For this review, take the finished solid that the model builds, in its own axes (mm). Face numbers are marked on the shaded views. A direction names the side the tool comes from. Round coordinates to 2 decimals unless told otherwise and drop trailing zeros. Write each loop counter-clockwise with the first axis right and the second up, starting at its lowest first coordinate (ties: lowest second). Pieces come first, ordered by that corner, then holes. Notation, with made-up numbers: (22.5, 83.5) -> (79.5, 83.5) arc R33 ccw to (79.5, 117.5) -> close; hole circle Ø6 at (73, 33.5). An arc over 180 degrees is marked (long way). Write each question's results on one line, items separated by ' | '. Start each with the question number.
Item 1: To check wall thickness, follow line 1 along Y through (x, z) = (12.5, 3.75); line 2 along Y through (x, z) = (97.5, 6); line 3 along Y through (x, z) = (165, 12.5). State the ranges of each line that lie inside material, in increasing order.
Item 2: Tool access review of the marked faces 5 and 6: name each direction out of +Z, -Z, +X, -X, +Y, -Y from which nothing blocks a thin tool from reaching the whole face with its end or side.
Item 3: Add section C-C (y = 10). State the section outline as (x, z) points, plus the area to 3 significant figures.
Item 4: Add section B-B (x = 111.5). State the section outline as (y, z) points, plus the area to 3 significant figures.
Item 5: Add section A-A (z = 14.5). State the section outline as (x, y) points.
Item 6: The part is to be moulded in two halves that separate along Y. For the marked faces 1, 2, 3 and 4, say which applies: +Y half, -Y half, draft (parallel to the pull), parting line (faces both ways), or undercut.
Item 7: Clearance check with flat-ended pins moving along their axes: pin 1 (2.5 mm diameter, centred on x = 12.5, y = -47.5, fed in from -Z); pin 2 (3 mm diameter, centred on x = 15.5, z = 12, fed in from +Y); pin 3 (7.5 mm diameter, centred on x = 13.5, y = -44.5, fed in from +Z); pin 4 (1 mm diameter, centred on x = 159, z = 2.5, fed in from +Y). State where each tip first meets the part, or that it passes through.
from build123d import *

# Parameters (mm, degrees)
PAD_DEPTH       = 18
FILLET_R        = 5
FILLET001_R     = 5
FILLET002_R     = 1
FILLET003_R     = 1
CHAMFER_SIZE    = 7
CHAMFER001_SIZE = 7
SKETCH001_W     = 15
SKETCH001_H     = 15
POCKET_DEPTH    = 10
SKETCH002_R     = 1
POCKET001_DEPTH = 8
SKETCH003_R     = 1
POCKET002_DEPTH = 8


with BuildPart() as part:
    # Sketch → Pad (new body)
    with BuildSketch(Plane.XY):
        Polygon((206.173076, -21.002959), (196.173076, -21.002959), (188.480768, -50), (0, 0), (7.692308, 28.997041), (-10, 28.997041), (-10, -69.999032), (206.173076, -69.999032), align=None)
    extrude(amount=PAD_DEPTH)

    # Fillet
    fillet_edges = [part.edges().sort_by_distance(p)[0] for p in [
        (7.692308, 28.997041, 9),
    ]]
    fillet(fillet_edges, radius=FILLET_R)

    # Fillet001
    fillet001_edges = [part.edges().sort_by_distance(p)[0] for p in [
        (196.173076, -21.002959, 9),
    ]]
    fillet(fillet001_edges, radius=FILLET001_R)

    # Fillet002
    fillet002_edges = [part.edges().sort_by_distance(p)[0] for p in [
        (206.173076, -21.002959, 9),
    ]]
    fillet(fillet002_edges, radius=FILLET002_R)

    # Fillet003
    fillet003_edges = [part.edges().sort_by_distance(p)[0] for p in [
        (-10, 28.997041, 9),
    ]]
    fillet(fillet003_edges, radius=FILLET003_R)

    # Chamfer
    chamfer_edges = [part.edges().sort_by_distance(p)[0] for p in [
        (0, 0, 9),
    ]]
    chamfer(chamfer_edges, length=CHAMFER_SIZE)

    # Chamfer001
    chamfer001_edges = [part.edges().sort_by_distance(p)[0] for p in [
        (188.480768, -50, 9),
    ]]
    chamfer(chamfer001_edges, length=CHAMFER001_SIZE)

    # Sketch001 → Pocket (cut)
    with BuildSketch(Plane.XY.offset(18)):
        with Locations((12.5, -47.499032)):
            Rectangle(SKETCH001_W, SKETCH001_H)
        with Locations((97.5, -47.499032)):
            Rectangle(SKETCH001_W, SKETCH001_H)
    extrude(amount=-POCKET_DEPTH, mode=Mode.SUBTRACT)

    # Sketch002 → Pocket001 (cut)
    with BuildSketch(Plane.XY.offset(8)):
        with Locations((12.5, -47.499032)):
            Circle(SKETCH002_R)
    extrude(amount=-POCKET001_DEPTH, mode=Mode.SUBTRACT)

    # Sketch003 → Pocket002 (cut)
    with BuildSketch(Plane.XY.offset(8)):
        with Locations((97.5, -47.499032)):
            Circle(SKETCH003_R)
    extrude(amount=-POCKET002_DEPTH, mode=Mode.SUBTRACT)


solid = part.part
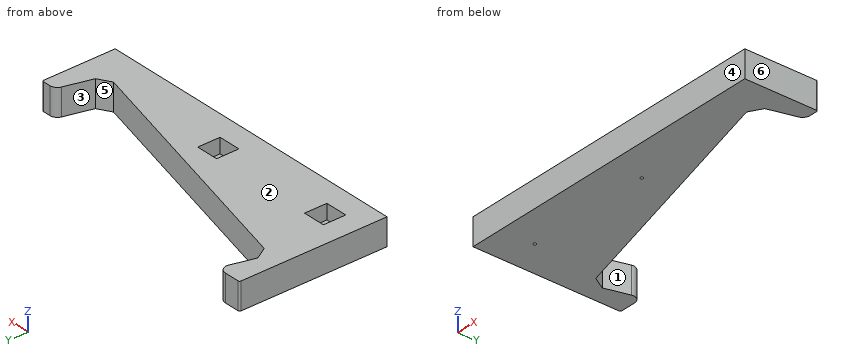
Responses:
1) line 1: y = -70 to -48.5, -46.5 to -3.32 | line 2: y = -70 to -48.5, -46.5 to -25.86 | line 3: y = -70 to -43.77
2) face 5: +Z, -Z, +Y | face 6: +Z, -Z, +X, +Y, -Y
3) outline: (-10, 0) -> (2.65, 0) -> (2.65, 18) -> (-10, 18) -> close | area: 228 mm^2
4) outline: (-70, 0) -> (-29.58, 0) -> (-29.58, 18) -> (-70, 18) -> close | area: 728 mm^2
5) outline: (-10, -70) -> (206.17, -70) -> (206.17, -22) arc R1 ccw to (205.17, -21) -> (200.02, -21) arc R5 ccw to (195.19, -24.72) -> (190.28, -43.23) -> (181.71, -48.21) -> (6.77, -1.79) -> (1.79, 6.77) -> (6.03, 22.71) arc R5 ccw to (1.19, 29) -> (-9, 29) arc R1 ccw to (-10, 28) -> close; hole (5, -55) -> (20, -55) -> (20, -40) -> (5, -40) -> close; hole (90, -55) -> (105, -55) -> (105, -40) -> (90, -40) -> close
6) face 1: undercut | face 2: draft | face 3: +Y half | face 4: -Y half
7) pin 1: stops at z = 0 | pin 2: stops at y = -3.71 | pin 3: stops at z = 8 | pin 4: stops at y = -42.05
